Drawing for the job (mm, zero at the part's lowest x, y, z). Round coordinates to 2 decimals unless told otherwise and drop trailing zeros. Loops run counter-clockwise (first coordinate to the right, second up) from the corner with the lowest first, then second, coordinate; pieces in that order, holes last.
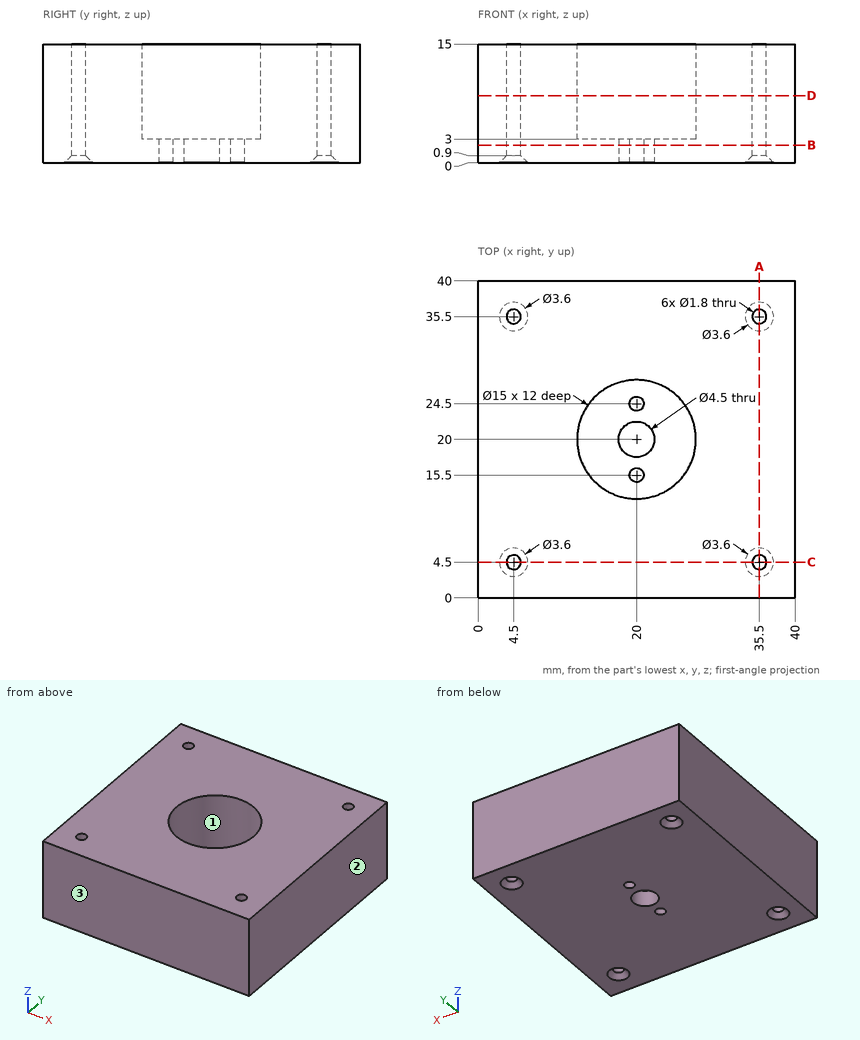
Q1. Pull direction Y, two halves, no side cores. Call the marked faces 1, 2 and 3: pulls with the +Y half, pulls with the -Y half, needs draft (parallel to the pull), parting line crosses it, or undercut.
Q2. Slice it at A-A on x = 35.5. Give the cut face in (y, z).
Q3. Probe line 1 (Y direction, x = 4.5, z = 9.5); line 2 (Y direction, x = 20, z = 2.2). List the from-to ranges inside material, lowest first.
Q4. Flat gauge pins, fed straight in: P1, Ø2.5, axis at x = 20, y = 20, coming from the +Z side; P2, Ø3, axis at x = 20, y = 15.5, coming from the +Z side. Where does each tip first touch, or does it go through?
Q5. Slice it at B-B on z = 2.25. Give the cut face in (x, y).
Q6. Slice it at D-D on z = 8.5. Give the cut face in (x, y).
Reply:
1. face 1: undercut
1. face 2: needs draft
1. face 3: pulls with the -Y half
2. outline: (0, 0) - (2.7, 0) - (3.6, 0.9) - (3.6, 15) - (0, 15) - close; (5.4, 0.9) - (6.3, 0) - (33.7, 0) - (34.6, 0.9) - (34.6, 15) - (5.4, 15) - close; (36.4, 0.9) - (37.3, 0) - (40, 0) - (40, 15) - (36.4, 15) - close
3. line 1: y = 0 to 3.6, 5.4 to 34.6, 36.4 to 40
3. line 2: y = 0 to 14.6, 16.4 to 17.75, 22.25 to 23.6, 25.4 to 40
4. P1: passes through
4. P2: stops at z = 3
5. outline: (0, 0) - (40, 0) - (40, 40) - (0, 40) - close; hole circle Ø1.8 at (4.5, 4.5); hole circle Ø1.8 at (4.5, 35.5); hole circle Ø4.5 at (20, 20); hole circle Ø1.8 at (20, 15.5); hole circle Ø1.8 at (20, 24.5); hole circle Ø1.8 at (35.5, 4.5); hole circle Ø1.8 at (35.5, 35.5)
6. outline: (0, 0) - (40, 0) - (40, 40) - (0, 40) - close; hole circle Ø1.8 at (4.5, 4.5); hole circle Ø1.8 at (4.5, 35.5); hole circle Ø15 at (20, 20); hole circle Ø1.8 at (35.5, 4.5); hole circle Ø1.8 at (35.5, 35.5)
